For this review, take the finished solid that the model builds, in its own axes (mm). A direction names the side the tool comes from. Give positions to 0.01 mm unless a question says otherwise; leave off trailing zeros. Write each loop counter-clockwise with the first axis right and the second up, starting at its lowest first coordinate (ties: lowest second). Pieces come first, ordered by that corner, then holes. Notation, with made-up numbers: M -6,16 L 33,16 A16 cw 33,26 Z; hole C -32.5,43 d1. An arc over 180 degrees is marked long. Answer as a JSON object with one key per item and string values. Group by question number.
```python
from build123d import *

# Parameters (mm, degrees)
SKETCH1_W               = 250
SKETCH1_H               = 200
BOSS_EXTRUDE1_DEPTH     = 20
BOSS_EXTRUDE2_START     = 65
SKETCH1_2_W             = 250
SKETCH1_2_H             = 200
BOSS_EXTRUDE2_DEPTH     = 20
SKETCH2_W               = 20
SKETCH2_H               = 20
BOSS_EXTRUDE3_DEPTH     = 45
SKETCH4_R               = 5
CUT_EXTRUDE1_DEPTH      = 10
SKETCH5_R               = 7.5
CUT_EXTRUDE2_DEPTH      = 75
CUT_EXTRUDE3_DEPTH      = 1
CUT_EXTRUDE3_DEPTH_BACK = 86
SKETCH7_R               = 7.5
CUT_EXTRUDE4_DEPTH      = 20
SKETCH8_W               = 160
SKETCH8_H               = 45
BOSS_EXTRUDE4_DEPTH     = 5


with BuildPart() as part:
    # Sketch1 → Boss-Extrude1 (new body)
    with BuildSketch(Plane(origin=(0, 0, 0), x_dir=(1, 0, 0), z_dir=(0, 1, 0))):
        Rectangle(SKETCH1_W, SKETCH1_H)
    extrude(amount=BOSS_EXTRUDE1_DEPTH)



with BuildPart() as body_2:
    # Sketch1<2> → Boss-Extrude2 (new body)
    with BuildSketch(Plane(origin=(0, 0, 0), x_dir=(1, 0, 0), z_dir=(0, 1, 0)).offset(BOSS_EXTRUDE2_START)):
        Rectangle(SKETCH1_2_W, SKETCH1_2_H)
    extrude(amount=BOSS_EXTRUDE2_DEPTH)


with BuildPart() as part_1:
    add(part.part)

    add(body_2.part)  # Boss-Extrude3 merges body 2
    # Sketch2 → Boss-Extrude3 (add)
    with BuildSketch(Plane(origin=(0, 20, 0), x_dir=(1, 0, 0), z_dir=(0, 1, 0))):
        with Locations((-115, -90)):
            Rectangle(SKETCH2_W, SKETCH2_H)
        with Locations((-115, 90)):
            Rectangle(SKETCH2_W, SKETCH2_H)
        with Locations((115, 90)):
            Rectangle(SKETCH2_W, SKETCH2_H)
        with Locations((115, -90)):
            Rectangle(SKETCH2_W, SKETCH2_H)
    extrude(amount=BOSS_EXTRUDE3_DEPTH)

    # Sketch4 → Cut-Extrude1 (cut)
    with BuildSketch(Plane(origin=(0, 85, 0), x_dir=(1, 0, 0), z_dir=(0, 1, 0))):
        with Locations((100, 0)):
            Circle(SKETCH4_R)
        with Locations((-100, -80)):
            Circle(SKETCH4_R)
        with Locations((-100, 80)):
            Circle(SKETCH4_R)
    extrude(amount=-CUT_EXTRUDE1_DEPTH, mode=Mode.SUBTRACT)

    # Sketch5 → Cut-Extrude2 (cut)
    with BuildSketch(Plane(origin=(0, 85, 0), x_dir=(1, 0, 0), z_dir=(0, 1, 0))):
        Circle(SKETCH5_R)
    extrude(amount=-CUT_EXTRUDE2_DEPTH, mode=Mode.SUBTRACT)

    # Sketch6 → Cut-Extrude3 (cut, two sides)
    with BuildSketch(Plane(origin=(0, 85, 0), x_dir=(1, 0, 0), z_dir=(0, 1, 0))) as cut_extrude3_sk:
        with BuildLine():
            Line((-125, 20), (-45, 20))
            ThreePointArc((-45, 20), (-25, 0), (-45, -20))
            Line((-45, -20), (-125, -20))
            Line((-125, -20), (-125, 20))
        make_face()
    extrude(amount=CUT_EXTRUDE3_DEPTH, mode=Mode.SUBTRACT)
    extrude(cut_extrude3_sk.sketch, amount=-CUT_EXTRUDE3_DEPTH_BACK, mode=Mode.SUBTRACT)

    # Sketch7 → Cut-Extrude4 (cut)
    with BuildSketch(Plane.XZ):
        with Locations((0, 50)):
            Circle(SKETCH7_R)
    extrude(amount=-CUT_EXTRUDE4_DEPTH, mode=Mode.SUBTRACT)

    # Sketch8 → Boss-Extrude4 (add)
    with BuildSketch(Plane(origin=(125, 0, 0), x_dir=(0, 0, -1), z_dir=(1, 0, 0))):
        with Locations((0, 42.5)):
            Rectangle(SKETCH8_W, SKETCH8_H)
    extrude(amount=-BOSS_EXTRUDE4_DEPTH)


solid = part_1.part
```
Item 1: Consider section D-D (x = -84.5). Give the boundary of the cut face in (y, z), plus the area to 3 significant figures.
Item 2: Consider section C-C (y = 46). Give the boundary of the cut face in (x, z).
Item 3: Machinability: for faces 4 (the flat face through (-86, 10, -20)), 5 (the flat face through (0, 10, 0)), 6 (the flat face through (120, 43, 1)), 7 (the flat face through (-105, 42, -90)), which of the approach directions +Z, -Z, +X, -X, +Y, -Y give a long, thin tool a straight path to every point of the face, cutting with its end or side? Answer none if there is none.
Item 4: Draft analysis for pull direction Y (two halves, no side actions). For faces 1 (the cylindrical face through (104.619, 80.07, 1.915)), 2 (the flat face through (-2, 85, -24)), 3 (the flat face through (-115, 42, 80)), state which applies: released by +Y, released by -Y, zero draft, split by the parting line, or undercut.
Item 5: To check wall thickness, follow probe 1 along X at (y, z) = (80.5, 0); probe 2 along Z at (x, y) = (0, 16); probe 3 along Z at (x, y) = (-100, 79.25). State the ranges of each line that lie inside material, in increasing order.
Item 6: Insertion check: P1, Ø5, axis at x = 98.5, z = -2.5, coming from the +Y side; P2, Ø4.5, axis at x = 0.5, z = -1.5, coming from the +Y side; P3, Ø3, axis at x = -98, z = -78, coming from the +Y side. Each pin has a flat end and moves straight along its axis. Give the tip position at first contact, or say it passes through.
Item 7: Consider section B-B (x = 100). Give the boundary of the cut face in (y, z), plus the area to 3 significant figures.
Item 8: Consider section A-A (z = 0). Give the boundary of the cut face in (x, y), plus the area to 4 significant figures.
Result set:
{
 "1": {"outline": "M 0,-100 L 20,-100 L 20,-20 L 0,-20 Z; M 0,20 L 20,20 L 20,100 L 0,100 Z; M 65,-100 L 85,-100 L 85,-20 L 65,-20 Z; M 65,20 L 85,20 L 85,100 L 65,100 Z", "area": "6,400 mm^2"},
 "2": {"outline": "M -125,-100 L -105,-100 L -105,-80 L -125,-80 Z; M -125,80 L -105,80 L -105,100 L -125,100 Z; M 105,-100 L 125,-100 L 125,100 L 105,100 L 105,80 L 120,80 L 120,-80 L 105,-80 Z"},
 "3": {"face 4": "-X, +Y, -Y", "face 5": "+Y", "face 6": "-X", "face 7": "+Z, -Z"},
 "4": {"face 1": "zero draft", "face 2": "released by +Y", "face 3": "undercut"},
 "5": {"probe 1": "x = -25 to -7.5, 7.5 to 95, 105 to 125", "probe 2": "z = -100 to -7.5, 7.5 to 42.5, 57.5 to 100", "probe 3": "z = -100 to -85, -75 to -20, 20 to 75, 85 to 100"},
 "6": {"P1": "stops at y = 85", "P2": "stops at y = 10", "P3": "stops at y = 75"},
 "7": {"outline": "M 0,-100 L 20,-100 L 20,100 L 0,100 Z; M 65,-100 L 85,-100 L 85,-5 L 75,-5 L 75,5 L 85,5 L 85,100 L 65,100 Z", "area": "7,900 mm^2"},
 "8": {"outline": "M -25,0 L 125,0 L 125,85 L 105,85 L 105,75 L 95,75 L 95,85 L 7.5,85 L 7.5,65 L 120,65 L 120,20 L 7.5,20 L 7.5,10 L -7.5,10 L -7.5,20 L -25,20 Z; M -25,65 L -7.5,65 L -7.5,85 L -25,85 Z", "area": "5,675 mm^2"}
}
